from build123d import *

# Parameters (mm, degrees)
F1_DEPTH  = 12.7
F3_DEPTH  = 2.778125
F5_D      = 3.5052
F5_DEPTH  = 19.05
F7_DEPTH  = 2.54
F8_R      = 10.16
F9_R      = 10.16
F10_R     = 2.54
F11_R     = 5.08
F13_R     = 1
F14_R     = 1
F16_D     = 3.5052
F16_DEPTH = 12.7
F17_DEPTH = 25


with BuildPart() as f1:
    # F0 (on Front) → F1 (new body)
    with BuildSketch(Plane.XZ):
        with BuildLine():
            Line((-6.35, 49.993444), (-6.35, 24.593444))
            Line((-6.35, 24.593444), (-6.798163, 24.473352))
            Line((-6.798163, 24.473352), (-57.404, 10.912781))
            Line((-57.404, 10.912781), (-57.404, 29.962781))
            Line((-57.404, 29.962781), (-62.484, 29.962781))
            Line((-62.484, 29.962781), (-62.484, 12.458641))
            Line((-62.484, 12.458641), (-62.484, 10.109072))
            ThreePointArc((-62.484, 10.109072), (-63.5, -10.16), (-64.516, 10.109072))
            Line((-64.516, 10.109072), (-64.516, 12.458641))
            Line((-64.516, 12.458641), (-64.516, 29.962781))
            Line((-64.516, 29.962781), (-69.596, 29.962781))
            Line((-69.596, 29.962781), (-69.596, 10.912781))
            ThreePointArc((-69.596, 10.912781), (-74.412781, -6.096), (-57.404, -10.912781))
            Line((-57.404, -10.912781), (-6.57485, -24.534289))
            ThreePointArc((-6.57485, -24.534289), (24.564124, -6.462493), (6.35, 24.593444))
            Line((6.35, 24.593444), (6.35, 49.993444))
            Line((6.35, 49.993444), (1.27, 49.993444))
            Line((1.27, 49.993444), (1.27, 25.36823))
            Line((1.27, 25.36823), (1.27, 20.280274))
            ThreePointArc((1.27, 20.280274), (0, -20.32), (-1.27, 20.280274))
            Line((-1.27, 20.280274), (-1.27, 25.36823))
            Line((-1.27, 25.36823), (-1.27, 49.993444))
            Line((-1.27, 49.993444), (-6.35, 49.993444))
        make_face()
    extrude(amount=F1_DEPTH)

    # F2 (on face) → F3 (cut)
    with BuildSketch(Plane.YZ.offset(6.35)):
        Polygon((-8.65969, 33.292944), (-4.04031, 33.292944), (-1.73062, 37.293444), (-4.04031, 41.293944), (-8.65969, 41.293944), (-10.96938, 37.293444), align=None)
    extrude(amount=-F3_DEPTH, mode=Mode.SUBTRACT)

    # F5
    with Locations(Plane.YZ.offset(3.571875)):
        with Locations((-6.35, 37.293444)):
            Hole(F5_D / 2, depth=F5_DEPTH)

    # F6 (on face) → F7 (cut)
    with BuildSketch(Plane.YZ.offset(-57.404)):
        Polygon((-11.067651, 20.437781), (-8.776292, 16.469031), (-4.193574, 16.469031), (-1.902215, 20.437781), (-4.193574, 24.406531), (-8.776292, 24.406531), align=None)
    extrude(amount=-F7_DEPTH, mode=Mode.SUBTRACT)

    # F8
    f8_edges = [f1.edges().sort_by_distance(p)[0] for p in [
        (-6.35, -6.35, 24.593444),
    ]]
    fillet(f8_edges, radius=F8_R)

    # F9
    f9_edges = [f1.edges().sort_by_distance(p)[0] for p in [
        (6.35, -6.35, 24.593444),
    ]]
    fillet(f9_edges, radius=F9_R)

    # F10
    f10_edges = [f1.edges().sort_by_distance(p)[0] for p in [
        (-57.404, -6.35, 10.912781),
    ]]
    fillet(f10_edges, radius=F10_R)

    # F11
    f11_edges = [f1.edges().sort_by_distance(p)[0] for p in [
        (-69.596, -6.35, 10.912781),
    ]]
    fillet(f11_edges, radius=F11_R)

    # F13
    f13_edges = [f1.edges().sort_by_distance(p)[0] for p in [
        (-63.5, -12.7, -10.16),
    ]]
    fillet(f13_edges, radius=F13_R)

    # F14
    f14_edges = [f1.edges().sort_by_distance(p)[0] for p in [
        (-63.5, 0, -10.16),
    ]]
    fillet(f14_edges, radius=F14_R)

    # F16
    with Locations(Plane.YZ.offset(-59.944)):
        with Locations((-6.35, 20.437781)):
            Hole(F16_D / 2, depth=F16_DEPTH)

    # F12 (on face) → F17 (cut)
    with BuildSketch(Plane.XZ.offset(12.7)):
        with BuildLine():
            ThreePointArc((-52.974038, 7.756792), (-49.845473, -0.719281), (-54.042015, -8.720579))
            Line((-54.042015, -8.720579), (-19.25646, -14.533902))
            ThreePointArc((-19.25646, -14.533902), (-25.435108, -0.999564), (-20.629572, 13.080949))
            Line((-20.629572, 13.080949), (-52.974038, 7.756792))
        make_face()
    extrude(amount=-F17_DEPTH, mode=Mode.SUBTRACT)


solid = f1.part
Design review of the part built by this model. Coordinates are the model's own, in mm. A direction names the side the tool comes from. Coordinates: 2 decimals unless noted, no trailing zeros. Write each loop counter-clockwise with the first axis right and the second up, starting at its lowest first coordinate (ties: lowest second). Pieces come first, ordered by that corner, then holes. Notation, with made-up numbers: (64.25, 4) - (122.25, 4) arc R23 ccw to (122.25, 23) - close; hole circle Ø3 at (42, -8.5). An arc over 180 degrees is marked (long way). Use one line per item in the form item = value.
Q1. Machinability: for faces 5 (the flat face through (-58.66, -3.03, 22.39)), 6 (the flat face through (-1.27, -6, 35)), 7 (the flat face through (-6.35, -6, 41)), which of the approach directions +Z, -Z, +X, -X, +Y, -Y give a long, thin tool a straight path to every point of the face, cutting with its end or side? Answer none if there is none.
Taken from the geometry:
face_5 = none
face_6 = +Z, +Y, -Y
face_7 = +Z, -X, +Y, -Y
Q2. The part is to be moulded in two halves that separate along Z. For faces 1 (the cylindrical face through (7.78, -6.44, 26.3)), 2 (the flat face through (-62.484, -6.3, 22.4)), 3 (the cylindrical face through (-67.092, -5.97, 18.727)), 4 (the flat face through (4.98, -2.9, 35.27)), say which applies: +Z half, -Z half, draft (parallel to the pull), parting line (faces both ways), or undercut.
Taken from the geometry:
face_1 = +Z half
face_2 = draft
face_3 = undercut
face_4 = undercut
Q3. Insertion check: pin 1 Ø3 at (y, z) = (-6.35, 37.29) entering from +X; pin 2 Ø2 at (x, y) = (-59, -5.5) entering from -Z; pin 3 Ø6.5 at (y, z) = (-5, 18.5) entering from +X; pin 4 Ø3 at (y, z) = (-3.5, -8) entering from -X. Each pin has a flat end and moves straight along its axis. Give the tip position at first contact, or say it passes through.
Taken from the geometry:
pin_1 = through
pin_2 = -12
pin_3 = 20.31
pin_4 = -74.18
Q4. Consider section B-B (x = -42). Write out the cut boundary in (y, z), plus the area to 3 significant figures.
Taken from the geometry:
outline = (-12.7, -15.04) - (0, -15.04) - (0, -10.73) - (-12.7, -10.73) - close; (-12.7, 9.56) - (0, 9.56) - (0, 15.04) - (-12.7, 15.04) - close
area = 124 mm^2
Q5. For probe 1 along X at (y, z) = (-9.25, 0); probe 2 along X at (y, z) = (-5.75, 40.5); probe 3 along X at (y, z) = (-9, 5.5), list the stretches that pass through material, from the lowest coordinate up.
Taken from the geometry:
probe_1 = -76 to -73.66, -53.34 to -49.82, -25.46 to -20.32, 20.32 to 25.4
probe_2 = -6.35 to -1.27, 1.27 to 3.57
probe_3 = -74.72 to -72.04, -54.96 to -51.28, -24.69 to -19.56, 19.56 to 24.8
Q6. Consider section D-D (x = 0). Write out the cut boundary in (y, z), plus the area to 3 significant figures.
Taken from the geometry:
outline = (-12.7, -25.4) - (0, -25.4) - (0, -20.32) - (-12.7, -20.32) - close
area = 64.5 mm^2
Q7. Consider section A-A (y = -6.35). Count the separate pieces of the cut face and the enclosed holes in it, plus the area to 3 significant figures.
Taken from the geometry:
separate_pieces = 5
enclosed_holes = 1
area = 1,670 mm^2
